Work out the finished part from the listing and answer in its coordinate system (mm). Coordinates: 2 decimals unless noted, no trailing zeros. Write each loop counter-clockwise with the first axis right and the second up, starting at its lowest first coordinate (ties: lowest second). Pieces come first, ordered by that corner, then holes. Notation, with made-up numbers: (61, -25) - (119, -25) arc R35 cw to (119, 12) - close; hole circle Ø10 at (88, 79). An arc over 180 degrees is marked (long way). Use one line per item in the form item = value. Start each with the question number.
Item 1: Consider probe 1 along Y at (x, z) = (0, -0.55); probe 2 along X at (y, z) = (1.25, 0.1); probe 3 along Z at (x, y) = (1.75, 0.25). Determine where each line is inside the solid, lowest interval first.
Item 2: A cutting plane is placed at A-A (y = 0). Write down the section's boundary in (x, z).
Item 3: Determine the mould class of faces 1 (the flat face through (-1, -2, -1.55)), 2 (the cylindrical face through (-1.5, 0.07, -0.02)), 3 (the cylindrical face through (3.233, -1.341, 0.16)) for opening direction Y: released by +Y, released by -Y, zero draft, split by the parting line, or undercut.
Item 4: Given pin 1 (1 mm diameter, centred on x = 1.5, z = 0, fed in from -Y), flat-ended and moving along its own axis, determine where the tip first touches the part or whether it passes through.
Item 5: A cutting plane is placed at C-C (z = 0.6). Write down the section's boundary in (x, y), then the cut area to 3 significant figures.
from build123d import *
from OCP.BRepFilletAPI import BRepFilletAPI_MakeChamfer

# Parameters (mm, degrees)
CROQUIS1_R              = 3.5
CROQUIS1_R_2            = 1.5
SALIENTE_EXTRUIR1_DEPTH = 1.5
CHAFL_N1_SIZE           = 0.4
CHAFL_N1_SIZE2          = 0.692820323
CROQUIS2_R              = 2.860932506
CROQUIS2_R_2            = 2.065541469
SALIENTE_EXTRUIR2_DEPTH = 1.55


with BuildPart() as part:
    # Croquis1 → Saliente-Extruir1 (new, symmetric)
    with BuildSketch(Plane.XY):
        Circle(CROQUIS1_R)
        Circle(CROQUIS1_R_2, mode=Mode.SUBTRACT)
    extrude(amount=SALIENTE_EXTRUIR1_DEPTH, both=True)

    # Chaflán1: one chamfer whose edges measure the first distance from different faces: ONE call of the kernel's chamfer builder (chamfer() names one face for all edges)
    chafl_n1_edges_1 = [part.edges().sort_by_distance(p)[0] for p in [
        (-3.5, 0, -1.5),
    ]]
    chafl_n1_side_1 = [part.faces().sort_by_distance(p)[0] for p in [
        (-3.401005051, 0, -1.5),
    ]]
    chafl_n1_edges_2 = [part.edges().sort_by_distance(p)[0] for p in [
        (-3.5, 0, 1.5),
    ]]
    chafl_n1_side_2 = [part.faces().sort_by_distance(p)[0] for p in [
        (-3.5, 0, 0),
    ]]
    chafl_n1 = BRepFilletAPI_MakeChamfer(part.part.solid().wrapped)
    for e in chafl_n1_edges_1:
        chafl_n1.Add(CHAFL_N1_SIZE, CHAFL_N1_SIZE2, e.wrapped, chafl_n1_side_1[0].wrapped)  # the first distance lies on this face
    for e in chafl_n1_edges_2:
        chafl_n1.Add(CHAFL_N1_SIZE, CHAFL_N1_SIZE2, e.wrapped, chafl_n1_side_2[0].wrapped)  # the first distance lies on this face
    add(Compound.cast(chafl_n1.Shape()), mode=Mode.REPLACE)

    # Croquis2 → Saliente-Extruir2 (add, symmetric)
    with BuildSketch(Plane(origin=(0, 0, 0), x_dir=(-1, 0, 0), z_dir=(0, 0, -1))):
        Circle(CROQUIS2_R)
        with Locations(Location((0, 0, 0), (0, 0, 180))):
            Circle(CROQUIS2_R_2, mode=Mode.SUBTRACT)
    extrude(amount=SALIENTE_EXTRUIR2_DEPTH, both=True)


solid = part.part
Answer:
q1.probe_1 = -3.5 to -1.5, 1.5 to 3.5
q1.probe_2 = -3.27 to -0.83, 0.83 to 3.27
q1.probe_3 = -1.5 to 1.5
q2.outline = (-3.5, -0.81) - (-3.1, -1.5) - (-2.86, -1.5) - (-2.86, -1.55) - (-2.07, -1.55) - (-2.07, -1.5) - (-1.5, -1.5) - (-1.5, 1.5) - (-2.07, 1.5) - (-2.07, 1.55) - (-2.86, 1.55) - (-2.86, 1.47) - (-3.5, 1.1) - close; (1.5, -1.5) - (2.07, -1.5) - (2.07, -1.55) - (2.86, -1.55) - (2.86, -1.5) - (3.1, -1.5) - (3.5, -0.81) - (3.5, 1.1) - (2.86, 1.47) - (2.86, 1.55) - (2.07, 1.55) - (2.07, 1.5) - (1.5, 1.5) - close
q3.face_1 = zero draft
q3.face_2 = undercut
q3.face_3 = split by the parting line
q4.pin_1 = -3.35
q5.outline = circle Ø7 at (0, 0); hole circle Ø3 at (0, 0)
q5.area = 31.4 mm²
